Verification items for the finished model (mm, model axes). Round coordinates to 2 decimals unless told otherwise and drop trailing zeros. Write each loop counter-clockwise with the first axis right and the second up, starting at its lowest first coordinate (ties: lowest second). Pieces come first, ordered by that corner, then holes. Notation, with made-up numbers: M -30.5,43.25 L -21.5,43.25 A14 ccw -21.5,59.25 Z; hole C -24.75,88.25 d11. An arc over 180 degrees is marked long. One line per item, written item: value. Start each with the question number.
Item 1: Thickness scan on probe 1 along Y at (x, z) = (11.75, 1.5); probe 2 along Y at (x, z) = (5.25, 2.25); probe 3 along Z at (x, y) = (5.25, 3). Record the ranges inside material, lowest first. Write a range as from..to.
Item 2: Gauge pin test, flat end, axial feed: pin 1 (6 mm diameter, centred on x = 6.5, y = 22, fed in from -Z). Record the tip position at first contact, or that the pin passes through.
Item 3: Section check B-B, the plane z = 4. Record the cut outline in (x, y).
Item 4: Section check C-C, the plane y = 1.5. Record the cut outline in (x, z), then the cut area to 3 significant figures.
Autodesk Inventor part; units mm, degrees
ref_plane "YZ Plane" through (0, 0, 0) normal (1, 0, 0) x (0, 1, 0)
ref_plane "XZ Plane" through (0, 0, 0) normal (0, 1, 0) x (-1, 0, 0)
ref_plane "XY Plane" through (0, 0, 0) normal (0, 0, 1) x (1, 0, 0)
sketch "Sketch1" plane through (0, 0, 0) normal (0, 0, 1) x (1, 0, 0)
  line L0 (0, 0) -> (19.05, 0)
  line L1 (19.05, 0) -> (19.05, 25.4)
  line L2 (19.05, 25.4) -> (0, 25.4)
  line L3 (0, 25.4) -> (0, 0)
  dimension "d0" = 19.05
  dimension "d1" = 25.4
extrude "Extrusion1" add sketch "Sketch1" along normal blind 6.35
fillet "Fillet1" radius 6.35 1 edges at (9.525, 0, 6.35)
properties part number "spacer_block" material "Acetal Resin, Black"
Response values:
1. probe 1: y = 0.18..25.4
1. probe 2: y = 0.41..25.4
1. probe 3: z = 0..5.39
2. pin 1: stops at z = 0
3. outline: M 0,1.42 L 19.05,1.42 L 19.05,25.4 L 0,25.4 Z
4. outline: M 0,0 L 19.05,0 L 19.05,4.1 L 0,4.1 Z
4. area: 78.1 mm2
